```python
from build123d import *

# Parameters (mm, degrees)
SKETCH1_W               = 42
SKETCH1_H               = 42
BOSS_EXTRUDE1_DEPTH     = 39
SKETCH2_R               = 11
BOSS_EXTRUDE2_DEPTH     = 2
SKETCH3_R               = 2.5
BOSS_EXTRUDE3_DEPTH     = 22
CHAMFER1_SIZE           = 3
SKETCH4_R               = 1.5
CUT_EXTRUDE1_DEPTH      = 10
CUT_EXTRUDE2_DEPTH      = 87.585218138
CUT_EXTRUDE2_DEPTH_BACK = 15


with BuildPart() as part:
    # Sketch1 → Boss-Extrude1 (new body)
    with BuildSketch(Plane.XY):
        with Locations((21, 21)):
            Rectangle(SKETCH1_W, SKETCH1_H)
    extrude(amount=BOSS_EXTRUDE1_DEPTH)

    # Sketch2 → Boss-Extrude2 (add)
    with BuildSketch(Plane.XY.offset(39)):
        with Locations((21, 21)):
            Circle(SKETCH2_R)
    extrude(amount=BOSS_EXTRUDE2_DEPTH)

    # Sketch3 → Boss-Extrude3 (add)
    with BuildSketch(Plane.XY.offset(41)):
        with Locations((21, 21)):
            Circle(SKETCH3_R)
    extrude(amount=BOSS_EXTRUDE3_DEPTH)

    # Chamfer1
    chamfer1_edges = [part.edges().sort_by_distance(p)[0] for p in [
        (0, 42, 19.5),
        (42, 42, 19.5),
        (42, 0, 19.5),
        (0, 0, 19.5),
    ]]
    chamfer(chamfer1_edges, length=CHAMFER1_SIZE)

    # Sketch4 → Cut-Extrude1 (cut)
    with BuildSketch(Plane.XY.offset(39)):
        with Locations((5.5, 36.5)):
            Circle(SKETCH4_R)
        with Locations((5.5, 5.5)):
            Circle(SKETCH4_R)
        with Locations((36.5, 5.5)):
            Circle(SKETCH4_R)
        with Locations((36.5, 36.5)):
            Circle(SKETCH4_R)
    extrude(amount=-CUT_EXTRUDE1_DEPTH, mode=Mode.SUBTRACT)

    # Sketch5 → Cut-Extrude2 (cut, two sides: drawn at the far end of the back side and taken through both)
    with BuildSketch(Plane.XY.offset(63).offset(-CUT_EXTRUDE2_DEPTH_BACK)):
        Polygon((23, 96.850602173), (23, 22.5), (23, 19.5), (23, -54.850602173), (171.701204346, -54.850602173), (171.701204346, 96.850602173), align=None)
    extrude(amount=CUT_EXTRUDE2_DEPTH + CUT_EXTRUDE2_DEPTH_BACK, mode=Mode.SUBTRACT)


solid = part.part
```
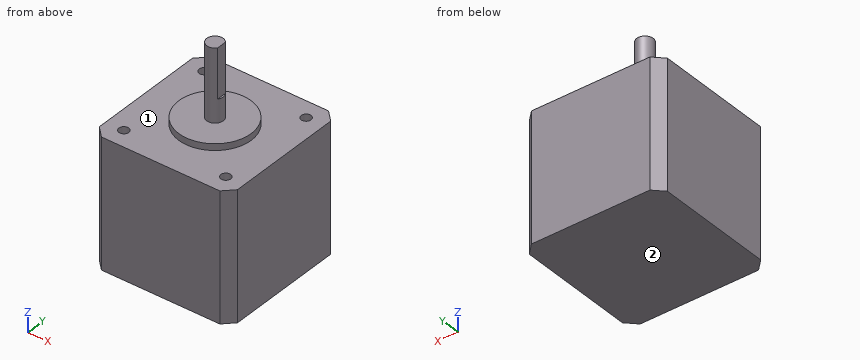
Geometry check sheet. Reference: the model listing, model coordinates, mm. Face numbers are marked on the shaded views. A direction names the side the tool comes from. Coordinates: 2 decimals unless noted, no trailing zeros. Write each loop counter-clockwise with the first axis right and the second up, starting at its lowest first coordinate (ties: lowest second). Pieces come first, ordered by that corner, then holes. Notation, with made-up numbers: M 16.25,-17.75 L 25.25,-17.75 A17 cw 25.25,-0.75 Z; hole C -19,1.25 d2. An arc over 180 degrees is marked long. One line per item, written item: value. Start each with the question number.
(1) Sectioned sample at A-A, the plane z = 36. Enter the section's corners in (x, y).
(2) Sectioned sample at B-B, the plane y = 36.5. Enter the section's corners in (x, z).
(3) Sectioned sample at C-C, the plane x = 21. Enter the section's corners in (y, z).
(4) Scan lines: line 1 along Y through (x, z) = (36.5, 36.25); line 2 along X through (y, z) = (5, 36); line 3 along Z through (x, y) = (21, 18). Record each from-to range of solid material in increasing order. Write a range as [from, to].
(5) Depth check by flat-ended pin: pin 1 (2.5 mm diameter, centred on x = 5.5, y = 5.5, fed in from -Z); pin 2 (2.5 mm diameter, centred on x = 36.5, y = 36.5, fed in from +Z); pin 3 (3.5 mm diameter, centred on x = 5, y = 36.5, fed in from +Z); pin 4 (1.5 mm diameter, centred on y = 21, z = 59, fed in from +X). Enter the tip coordinate at first touch or a pass-through.
(6) Sectioned sample at D-D, the plane y = 16.5. Enter the section's corners in (x, z), and give its area (3 significant figures).
(7) Tool access check on the marked faces 1 and 2. Record the directions out of +Z, -Z, +X, -X, +Y, -Y that give a thin tool (end or side, any length) a straight path to the whole face; none if there is none.
Filled sheet:
1. outline: M 0,3 L 3,0 L 39,0 L 42,3 L 42,39 L 39,42 L 3,42 L 0,39 Z; hole C 5.5,5.5 d3; hole C 5.5,36.5 d3; hole C 36.5,5.5 d3; hole C 36.5,36.5 d3
2. outline: M 0,0 L 42,0 L 42,39 L 38,39 L 38,29 L 35,29 L 35,39 L 7,39 L 7,29 L 4,29 L 4,39 L 0,39 Z
3. outline: M 0,0 L 42,0 L 42,39 L 32,39 L 32,41 L 23.5,41 L 23.5,63 L 18.5,63 L 18.5,41 L 10,41 L 10,39 L 0,39 Z
4. line 1: [0, 4], [7, 35], [38, 42]
4. line 2: [0, 4.09], [6.91, 35.09], [37.91, 42]
4. line 3: [0, 41]
5. pin 1: z = 0
5. pin 2: z = 29
5. pin 3: z = 39
5. pin 4: x = 23
6. outline: M 0,0 L 42,0 L 42,39 L 31.04,39 L 31.04,41 L 10.96,41 L 10.96,39 L 0,39 Z
6. area: 1,680 mm²
7. face 1: +Z
7. face 2: -Z, +X, -X, +Y, -Y
